Autodesk Inventor part; units mm, degrees
ref_plane "YZ Plane" through (0, 0, 0) normal (1, 0, 0) x (0, 1, 0)
ref_plane "XZ Plane" through (0, 0, 0) normal (0, 1, 0) x (-1, 0, 0)
ref_plane "XY Plane" through (0, 0, 0) normal (0, 0, 1) x (1, 0, 0)
sketch "スケッチ1" plane through (0, 0, 0) normal (0, 0, 1) x (1, 0, 0)
  line L0 (-27.5, 25) -> (27.5, 25)
  line L1 (27.5, 25) -> (27.5, 0)
  line L2 (27.5, 0) -> (-27.5, 0)
  line L3 (-27.5, 0) -> (-27.5, 25)
  line L4 (-27.5, 0) -> (27.5, 0)
  line L5 (27.5, 0) -> (27.5, -5)
  line L6 (27.5, -5) -> (-27.5, -5)
  line L7 (-27.5, -5) -> (-27.5, 0)
  circle A0 centre (-22.5, 15) radius 1.25
  line L8 (-27.3778, 15) -> (27.6222, 15)
  line L9 (0, 25) -> (0, -5)
  circle A1 centre (22.5, 15) radius 1.25
  point P0 (0, 0)
  point P1 (0, 0)
  point P2 (0, 0)
  dimension "d0" = 25
  dimension "d1" = 55
  dimension "d2" = 5
  dimension "d4" = 22.5
  dimension "d5" = 2.5
  dimension "d17" = 10
extrude "押し出し1" add sketch "スケッチ1" along normal blind 5 contours L0 L9 L2 L3 | L0 L1 L8 A1 L9 | L8 A1 L1 L2 L9
extrude "押し出し2" add sketch "スケッチ1" along normal blind 35 contours L2 L9 L6 L7 | L2 L5 L6 L9
sketch "スケッチ2" plane through (-27.5, -5, 0) normal (0, -1, 0) x (1, 0, 0)
  line L0 (0, 35) -> (55, 35)
  line L1 (54.9263, 23) -> (-0.0737, 23)
  line L2 (27.5, 35) -> (27.5, 0)
  circle A0 centre (27.5, 23) radius 3.15
  dimension "d15" = 6.3
  dimension "d18" = 12
extrude "押し出し3" cut sketch "スケッチ2" against normal blind 30
fillet "フィレット1" radius 3 2 edges at (0, -5, 0) (0, 0, 5)
fillet "フィレット2" radius 3 4 edges at (27.5, -2.5, 35) (-27.5, -2.5, 35) (27.5, 25, 2.5) (-27.5, 25, 2.5)
equation "\"BendRadius\" = Thickness"
equation "\"BendReliefWidth\" = Thickness"
equation "\"BendReliefDepth\" = 0.5 * Thickness"
equation "\"CornerReliefSize\" = 4 * Thickness"
equation "\"MinimumRemnant\" = 2 * Thickness"
equation "\"TransitionRadius\" = BendRadius"
equation "\"JacobiRadiusSize\" = BendRadius"
equation "\"GapSize\" = Thickness"
Can you work these out from the model? Positions are in its coordinate system, mm. A direction names the side the tool comes from. Give positions to 0.01 mm unless a question says otherwise; leave off trailing zeros. Write each loop counter-clockwise with the first axis right and the second up, starting at its lowest first coordinate (ties: lowest second). Pieces come first, ordered by that corner, then holes. Notation, with made-up numbers: M 65.25,66 L 84.25,66 A21 ccw 84.25,77 Z; hole C 5.25,19.25 d4. An arc over 180 degrees is marked long. Answer in a Markdown table with one row per item. Add a question column.
Item 1: Imagine slicing it at A-A, the plane x = 0. Write out the boundary of the cut face in (y, z), plus the area to 4 significant figures.
Item 2: For pin 1 Ø12 at (x, z) = (-2.5, 24) entering from +Y; pin 2 Ø2 at (x, y) = (22.5, 15) entering from -Z; pin 3 Ø5 at (x, y) = (20, 3) entering from +Z, each with a flat end and sliding along its axis, tell me the tip position at first contact or that it passes through.
Item 3: Imagine slicing it at B-B, the plane y = 15. Write out the boundary of the cut face in (x, z), plus the area to 3 significant figures.
Item 4: Please list where these lines run through material, in increasing order: L1, parallel to X at y = 15, z = 1.3; L2, parallel to X at y = -1.35, z = 23; L3, parallel to Z at x = 0, y = -1.6.
Item 5: Imagine slicing it at C-C, the plane x = -16.5. Write out the boundary of the cut face in (y, z), plus the area to 3 significant figures.
Item 6: Imagine slicing it at D-D, the plane z = 24.5. Write out the boundary of the cut face in (x, y), plus the area to 3 significant figures.
Item 7: On a 3-axis mill with a long thin cutter (end or side, diameter ignored), from which of +Z, -Z, +X, -X, +Y, -Y can I reach the whole of each face in a straight line? I mean faces 4 (the flat face through (0, 14, 5)), 5 (the flat face through (0, -5, 19)). Say none if no direction works.
Item 8: We'd pull the mould along Y, two halves only. Please class faces 1 (the cylindrical face through (-21.828, 13.946, 2.465)), 2 (the cylindrical face through (26.64, 24.1, 2.54)), 3 (the flat face through (0, 12, 0)): released by +Y, released by -Y, zero draft, split by the parting line, or undercut.
Evaluation:
| question | item | result |
|---|---|---|
| 1 | outline | M -5,3 A3 ccw -2,0 L 25,0 L 25,5 L 3,5 A3 cw 0,8 L 0,19.85 L -5,19.85 Z; M -5,26.15 L 0,26.15 L 0,35 L -5,35 Z |
| 1 | area | 268.5 mm² |
| 2 | pin 1 | stops at y = 0 |
| 2 | pin 2 | passes through |
| 2 | pin 3 | stops at z = 6.34 |
| 3 | outline | M -27.5,0 L -23.75,0 L -23.75,5 L -27.5,5 Z; M -21.25,0 L 21.25,0 L 21.25,5 L -21.25,5 Z; M 23.75,0 L 27.5,0 L 27.5,5 L 23.75,5 Z |
| 3 | area | 250 mm² |
| 4 | L1 | x = -27.5 to -23.75, -21.25 to 21.25, 23.75 to 27.5 |
| 4 | L2 | x = -27.5 to -3.15, 3.15 to 27.5 |
| 4 | L3 | z = 0 to 19.85, 26.15 to 35 |
| 5 | outline | M -5,3 A3 ccw -2,0 L 25,0 L 25,5 L 3,5 A3 cw 0,8 L 0,35 L -5,35 Z |
| 5 | area | 300 mm² |
| 6 | outline | M -27.5,-5 L -2.77,-5 L -2.77,0 L -27.5,0 Z; M 2.77,-5 L 27.5,-5 L 27.5,0 L 2.77,0 Z |
| 6 | area | 247 mm² |
| 7 | face 4 | +Z, +X, -X, +Y |
| 7 | face 5 | +Z, -Z, +X, -X, -Y |
| 8 | face 1 | undercut |
| 8 | face 2 | released by +Y |
| 8 | face 3 | zero draft |
